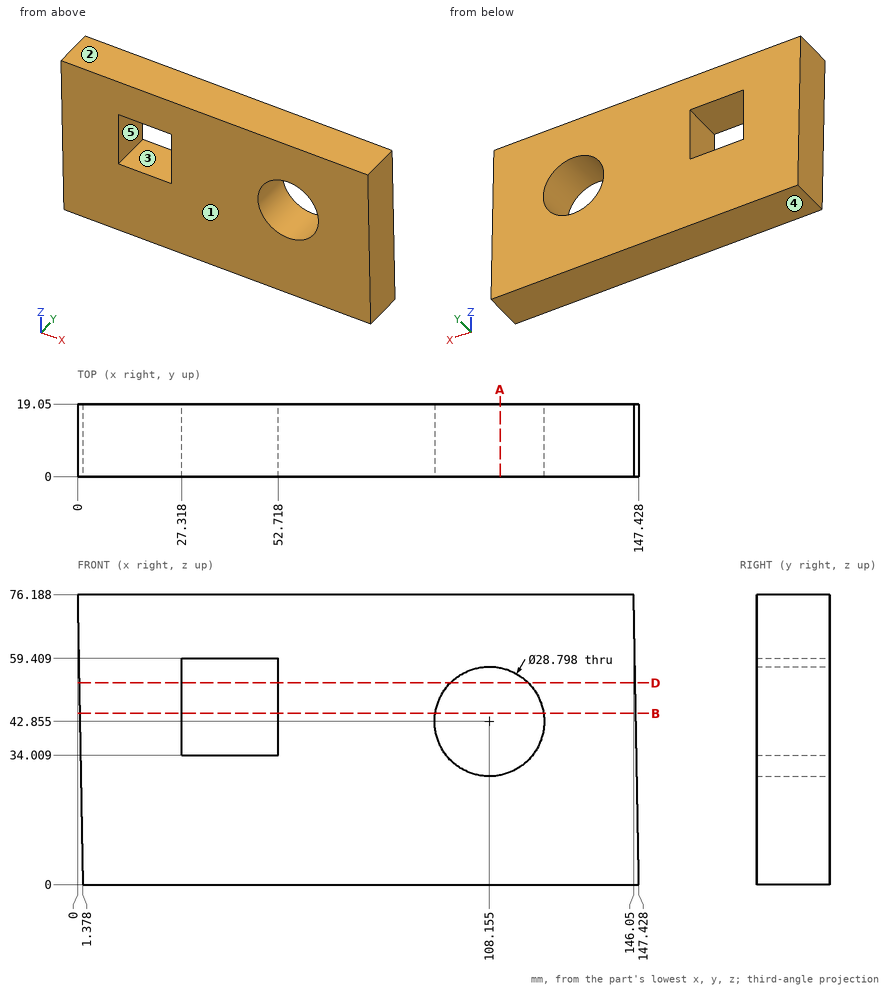
For this review, use the dimensioned drawing (mm, ordinates from the lowest corner) and the shaded views. A direction names the side the tool comes from. Give positions to 0.01 mm unless a question says otherwise; leave off trailing zeros. Write each loop counter-clockwise with the first axis right and the second up, starting at its lowest first coordinate (ties: lowest second). Pieces come first, ordered by that corner, then holes. Notation, with made-up numbers: M -33,38.5 L -5,38.5 A14 ccw -5,49.5 Z; hole C 63.5,76.25 d5. An arc over 180 degrees is marked long. Answer as a JSON object with one key per item and string values. Group by question number.
Item 1: Consider section D-D on z = 53. Write out the cut boundary in (x, y).
Item 2: Tool access review of the marked faces 4 and 5: name each direction out of +Z, -Z, +X, -X, +Y, -Y from which nothing blocks a thin tool from reaching the whole face with its end or side.
Item 3: Consider section A-A on x = 111. Write out the cut boundary in (y, z).
Item 4: Consider section B-B on z = 45. Count the separate pieces of the cut face and the enclosed holes in it, plus the area to 3 significant figures.
Item 5: For pin 1 Ø6 at (y, z) = (4, 58) entering from +X; pin 2 Ø23 at (x, z) = (108.15, 42.86) entering from -Y, all flat-tipped, find the tip position at first contact; note any pin that passes through.
Item 6: Draft analysis for pull direction Z (two halves, no side actions). For the marked faces 1, 2 and 3, state which applies: +Z half, -Z half, draft (parallel to the pull), parting line (faces both ways), or undercut.
Item 7: For probe 1 along X at (y, z) = (10.25, 47.5) (1 decimal); probe 2 along X at (y, z) = (16.25, 41) (1 decimal); probe 3 along Z at (x, y) = (29.5, 4), list the stretches that pass through material, from the lowest coordinate up. Write a range as [from, to].
Check result:
{
 "1": {"outline": "M 0.42,0 L 27.32,0 L 27.32,19.05 L 0.42,19.05 Z; M 52.72,0 L 97.94,0 L 97.94,19.05 L 52.72,19.05 Z; M 118.37,0 L 146.47,0 L 146.47,19.05 L 118.37,19.05 Z"},
 "2": {"face 4": "-Z, +X, -X, +Y, -Y", "face 5": "+Y, -Y"},
 "3": {"outline": "M 0,0 L 19.05,0 L 19.05,28.74 L 0,28.74 Z; M 0,56.97 L 19.05,56.97 L 19.05,76.19 L 0,76.19 Z"},
 "4": {"separate pieces": "3", "enclosed holes": "0", "area": "1,760 mm^2"},
 "5": {"pin 1": "stops at x = 146.43", "pin 2": "passes through"},
 "6": {"face 1": "draft", "face 2": "+Z half", "face 3": "undercut"},
 "7": {"probe 1": "x = [0.5, 27.3], [52.7, 94.5], [121.8, 146.6]", "probe 2": "x = [0.6, 27.3], [52.7, 93.9], [122.4, 146.7]", "probe 3": "z = [0, 34.01], [59.41, 76.19]"}
}
